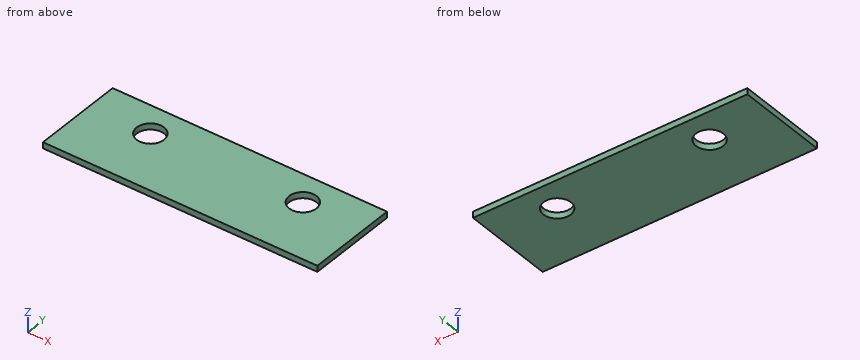
Autodesk Inventor part; units mm, degrees
ref_plane "YZ Plane" through (0, 0, 0) normal (1, 0, 0) x (0, 1, 0)
ref_plane "XZ Plane" through (0, 0, 0) normal (0, 1, 0) x (-1, 0, 0)
ref_plane "XY Plane" through (0, 0, 0) normal (0, 0, 1) x (1, 0, 0)
sketch "Sketch1" plane through (0, 0, 0) normal (0, 0, 1) x (1, 0, 0)
  line L0 (0, -3.4) -> (45, -3.4)
  line L1 (45, -3.4) -> (45, 11.6)
  line L2 (45, 11.6) -> (0, 11.6)
  line L3 (0, 11.6) -> (0, -3.4)
  point P0 (0, 0)
  dimension "d1" = 3.4
  dimension "d2" = 45
  dimension "d3" = 45
  dimension "d4" = 15
extrude "Plate1" add sketch "Sketch1" along normal blind 1
sketch "Sketch2" plane through (0, 0, 1) normal (0, 0, 1) x (1, 0, 0)
  line L0 (45, -3.4) -> (0, -3.4)
  line L1 (45, 11.6) -> (45, -3.4)
  line L2 (0, -3.4) -> (0, 11.6)
  point P0 (0, 0)
  point P1 (35, 6.6)
  point P2 (10, 6.6)
  dimension "d5" = 10
  dimension "d6" = 10
  dimension "d7" = 10
hole "Hole1" at (35, 6.6, 1) at (10, 6.6, 1) direction (0, 0, -1) diameter 4.5 end through all
equation "\"d13\" = Thickness"
equation "\"d0\" = Thickness"
equation "\"BendRadius\" = Thickness"
equation "\"BendReliefWidth\" = Thickness"
equation "\"BendReliefDepth\" = 0.5 * Thickness"
equation "\"CornerReliefSize\" = 4 * Thickness"
equation "\"MinimumRemnant\" = 2 * Thickness"
equation "\"TransitionRadius\" = BendRadius"
equation "\"JacobiRadiusSize\" = BendRadius"
equation "\"GapSize\" = Thickness"
properties part number "Pletina Terminal V2" material "Steel, Carbon"
Geometry: final body of the model. Coordinates: model frame, mm. Coordinates: 2 decimals unless noted, no trailing zeros. Order: outer loops, then holes, each group sorted by start corner. A loop starts at its lowest first (then second) coordinate and runs counter-clockwise, first axis right, second up. Notation, with made-up numbers: (12.5, -28.75) - (32.5, -28.75) arc R21 cw to (32.5, -6.75) - close; hole circle Ø4 at (59, 37). An arc over 180 degrees is marked (long way). Write each question's results on one line, items separated by ' | '.
1) Section B-B, the plane y = 6.6. Return loops of the section in (x, z).
Results list:
outline: (0, 0) - (7.75, 0) - (7.75, 1) - (0, 1) - close; (12.25, 0) - (32.75, 0) - (32.75, 1) - (12.25, 1) - close; (37.25, 0) - (45, 0) - (45, 1) - (37.25, 1) - close
2) Section A-A, the plane x = 10. Return loops of the section in (y, z), plus the area to 3 significant figures.
Results list:
outline: (-3.4, 0) - (4.35, 0) - (4.35, 1) - (-3.4, 1) - close; (8.85, 0) - (11.6, 0) - (11.6, 1) - (8.85, 1) - close | area: 10.5 mm^2
3) Section C-C, the plane z = 0.35. Return loops of the section in (x, y), plus the area to 3 significant figures.
Results list:
outline: (0, -3.4) - (45, -3.4) - (45, 11.6) - (0, 11.6) - close; hole circle Ø4.5 at (10, 6.6); hole circle Ø4.5 at (35, 6.6) | area: 643 mm^2
4) Pin query (flat end, axial travel): pin 1 (2.5 mm diameter, centred on x = 35, y = 6.6, fed in from -Z). Return the tip coordinate at first contact, or that it passes through.
Results list:
pin 1: through
5) Line query: line 1 (X direction, y = 6.6, z = 0.75); line 2 (Y direction, x = 10, z = 0.6); line 3 (Y direction, x = 37, z = 0.55). Output: solid intervals per line, ascending. Write a range as from..to.
Results list:
line 1: 0..7.75, 12.25..32.75, 37.25..45 | line 2: -3.4..4.35, 8.85..11.6 | line 3: -3.4..5.57, 7.63..11.6
